Input: part model. Units: mm. Frame: model coordinates. Face numbers are marked on the shaded views. A direction names the side the tool comes from. Coordinates: 2 decimals unless noted, no trailing zeros. Order: outer loops, then holes, each group sorted by start corner. A loop starts at its lowest first (then second) coordinate and runs counter-clockwise, first axis right, second up.
from build123d import *

# Parameters (mm, degrees)
F0_R          = 15
F1_DEPTH      = 18
F2_R          = 15
F3_DEPTH      = 5
F4_R          = 15
F5_DEPTH      = 5
F7_R          = 20
F8_DEPTH      = 14
F8_DEPTH_BACK = 14
F6_R          = 7
F9_DEPTH      = 20.001
F9_DEPTH_BACK = 20.001


with BuildPart() as f1:
    # F0 (on Top) → F1 (new body, symmetric)
    with BuildSketch(Plane.XY):
        Circle(F0_R)
    extrude(amount=F1_DEPTH, both=True)

    # F2 (on face) → F3 (join)
    with BuildSketch(Plane.XY.offset(18)):
        Circle(F2_R)
    extrude(amount=F3_DEPTH)

    # F4 (on face) → F5 (join)
    with BuildSketch(Plane(origin=(0, 0, -18), x_dir=(1, 0, 0), z_dir=(0, 0, -1))):
        Circle(F4_R)
    extrude(amount=F5_DEPTH)

    # F7 (on Top) → F8 (join, two sides)
    with BuildSketch(Plane.XY) as f8_sk:
        Circle(F7_R)
    extrude(amount=F8_DEPTH)
    extrude(f8_sk.sketch, amount=-F8_DEPTH_BACK)

    # F6 (on Right) → F9 (cut, two sides)
    with BuildSketch(Plane.YZ) as f9_sk:
        Circle(F6_R)
    extrude(amount=-F9_DEPTH, mode=Mode.SUBTRACT)
    extrude(f9_sk.sketch, amount=F9_DEPTH_BACK, mode=Mode.SUBTRACT)


solid = f1.part
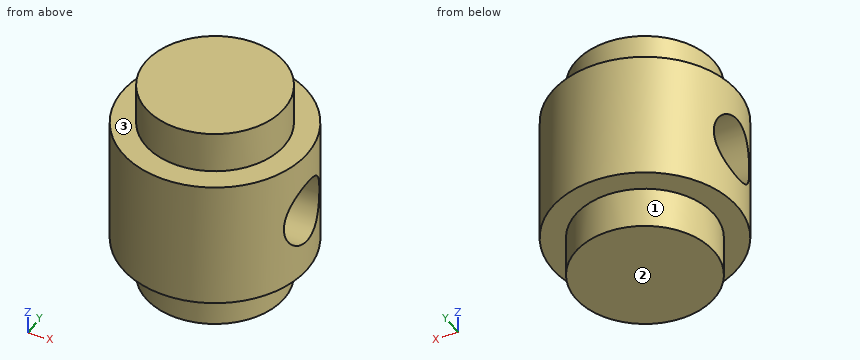
Item 1: Cut plane B-B on x = 2. Return loops of the section in (y, z).
Response values:
outline: (-19.9, -14) - (-14.87, -14) - (-14.87, -23) - (14.87, -23) - (14.87, -14) - (19.9, -14) - (19.9, 14) - (14.87, 14) - (14.87, 23) - (-14.87, 23) - (-14.87, 14) - (-19.9, 14) - close; hole circle Ø14 at (0, 0)
Item 2: Ray query, probe 1 along Z at (x, y) = (7.75, 0); probe 2 along Y at (x, z) = (-15, -0.5); probe 3 along Y at (x, z) = (-17.5, -1). Return the intervals inside material, ascending.
Response values:
probe 1: z = -23 to -7, 7 to 23
probe 2: y = -13.23 to -6.98, 6.98 to 13.23
probe 3: y = -9.68 to -6.93, 6.93 to 9.68
Item 3: Pin query (flat end, axial travel): pin 1 Ø12 at (y, z) = (-12.5, 9.5) entering from +X; pin 2 Ø8 at (x, z) = (-12, -4.5) entering from +Y; pin 3 Ø22.5 at (y, z) = (0, 0) entering from -X; pin 4 Ø2 at (x, z) = (4.5, -7) entering from -Y. Return the tip coordinate at first contact, or that it passes through.
Response values:
pin 1: stops at x = 18.91
pin 2: stops at y = 18.33
pin 3: stops at x = -20
pin 4: stops at y = -19.69
Item 4: Cut plane C-C on z = 19. Return loops of the section in (x, y).
Response values:
outline: circle Ø30 at (0, 0)
Item 5: Cut plane D-D on y = 10. Return loops of the section in (x, z).
Response values:
outline: (-17.32, -14) - (-11.18, -14) - (-11.18, -23) - (11.18, -23) - (11.18, -14) - (17.32, -14) - (17.32, 14) - (11.18, 14) - (11.18, 23) - (-11.18, 23) - (-11.18, 14) - (-17.32, 14) - close
Item 6: Cut plane A-A on y = 1.5. Return loops of the section in (x, z).
Response values:
outline: (-19.94, -14) - (-14.92, -14) - (-14.92, -23) - (14.92, -23) - (14.92, -14) - (19.94, -14) - (19.94, -6.84) - (-19.94, -6.84) - close; (-19.94, 6.84) - (19.94, 6.84) - (19.94, 14) - (14.92, 14) - (14.92, 23) - (-14.92, 23) - (-14.92, 14) - (-19.94, 14) - close
Item 7: Access query for the marked faces 1, 2 and 3. Directions: +Z, -Z, +X, -X, +Y, -Y. A direction counts if a zero-diameter tool reaches every point of the face in a straight line with its end or side. Return the directions, or none.
Response values:
face 1: -Z
face 2: -Z, +X, -X, +Y, -Y
face 3: +Z
